The listing builds one solid part. Answer for the finished solid, in the listing's coordinates (mm). A direction names the side the tool comes from. Give positions to 0.01 mm unless a question says otherwise; leave off trailing zeros. Write each loop counter-clockwise with the first axis right and the second up, starting at its lowest first coordinate (ties: lowest second). Pieces come first, ordered by that corner, then holes.
```python
from build123d import *

# Parameters (mm, degrees)
SKETCH2_R           = 20
SKETCH2_R_2         = 10
BOSS_EXTRUDE1_DEPTH = 26
SKETCH3_W           = 50.5
SKETCH3_H           = 100
BOSS_EXTRUDE2_DEPTH = 50
SKETCH6_W           = 19
SKETCH6_H           = 19
CUT_EXTRUDE1_DEPTH  = 129.115426472
CUT_EXTRUDE5_DEPTH  = 105.049267177
CUT_EXTRUDE6_DEPTH  = 105.049267177


with BuildPart() as part:
    # Sketch2 → Boss-Extrude1 (new body)
    with BuildSketch(Plane(origin=(0, 0, 0), x_dir=(0, 0, -1), z_dir=(1, 0, 0))):
        with Locations(Location((0, 0, 0), (0, 0, 180))):
            Circle(SKETCH2_R)
        with Locations(Location((0, 0, 0), (0, 0, 180))):
            Circle(SKETCH2_R_2, mode=Mode.SUBTRACT)
    extrude(amount=BOSS_EXTRUDE1_DEPTH)

    # Sketch3 → Boss-Extrude2 (add)
    with BuildSketch(Plane(origin=(26, 0, 0), x_dir=(0, 0, -1), z_dir=(1, 0, 0))):
        Rectangle(SKETCH3_W, SKETCH3_H)
    extrude(amount=BOSS_EXTRUDE2_DEPTH)

    # Sketch6 → Cut-Extrude1 (cut, through all)
    with BuildSketch(Plane.XZ.offset(50)):
        with Locations((35.5, 0)):
            Rectangle(SKETCH6_W, SKETCH6_H)
    extrude(amount=-CUT_EXTRUDE1_DEPTH, mode=Mode.SUBTRACT)

    # Sketch7 → Cut-Extrude5 (cut, through all)
    with BuildSketch(Plane(origin=(0, 0, -25.25), x_dir=(-1, 0, 0), z_dir=(0, 0, -1))):
        Polygon((-60, 50), (-26, 50), (-26, 35.294942904), align=None)
        Polygon((-60, -50), (-26, -35.294942904), (-26, -50), align=None)
    extrude(amount=-CUT_EXTRUDE5_DEPTH, mode=Mode.SUBTRACT)

    # Sketch9 → Cut-Extrude6 (cut, through all)
    with BuildSketch(Plane(origin=(0, 0, -25.25), x_dir=(-1, 0, 0), z_dir=(0, 0, -1))):
        Polygon((-76, 19.807249774), (-76, -25.192750226), (-61.483507586, -12), (-61.483507586, 12), align=None)
    extrude(amount=-CUT_EXTRUDE6_DEPTH, mode=Mode.SUBTRACT)


solid = part.part
```
Item 1: Each of these flat-tipped pins is pushed along its axis until it touches: P1, Ø4, axis at x = 47.5, z = -3, coming from the +Y side; P2, Ø6, axis at x = 21, y = -13.5, coming from the -Z side; P3, Ø5, axis at x = 43, z = 16, coming from the +Y side. Where does it stop, or does it pass through?
Conclusion:
P1: stops at y = 45.46
P2: stops at z = -17.02
P3: stops at y = 43.73
Item 2: A cutting plane is placed at A-A, the plane z = 0. Give the vertices of the cut face in (x, y).
Conclusion:
outline: (0, -20) - (26, -20) - (26, -10) - (0, -10) - close; (0, 10) - (26, 10) - (26, 20) - (0, 20) - close; (45, -43.51) - (60, -50) - (76, -50) - (76, -25.19) - (61.48, -12) - (61.48, 12) - (76, 19.81) - (76, 50) - (60, 50) - (45, 43.51) - close
Item 3: A cutting plane is placed at C-C, the plane y = 0. Give the vertices of the cut face in (x, z), plus the area to 3 significant figures.
Conclusion:
outline: (0, -20) - (26, -20) - (26, -25.25) - (61.48, -25.25) - (61.48, 25.25) - (26, 25.25) - (26, 20) - (0, 20) - (0, 10) - (26, 10) - (26, 9.5) - (45, 9.5) - (45, -9.5) - (26, -9.5) - (26, -10) - (0, -10) - close
area: 1,950 mm2
Item 4: Determine the mould class of faces 5 (the face through (45, -1, 0)), 6 (the face through (68.64, 15.85, -0.35)), 7 (the face through (68, 50, 0)) for opening direction Y: pulls with the +Y half, pulls with the -Y half, needs draft (parallel to the pull), parting line crosses it, or undercut.
Conclusion:
face 5: needs draft
face 6: undercut
face 7: pulls with the +Y half
Item 5: A cutting plane is placed at B-B, the plane x = 27.5. Give the vertices of the cut face in (y, z), plus the area to 3 significant figures.
Conclusion:
outline: (-35.94, -25.25) - (35.94, -25.25) - (35.94, -9.5) - (-35.94, -9.5) - close; (-35.94, 9.5) - (35.94, 9.5) - (35.94, 25.25) - (-35.94, 25.25) - close
area: 2,260 mm2
Item 6: Consider probe 1 along Y at (x, z) = (13, 0); probe 2 along Z at (x, y) = (42, 39.5); probe 3 along X at (y, z) = (-28.5, 8). Determine where each line is inside the solid, lowest interval first.
Conclusion:
probe 1: y = -20 to -10, 10 to 20
probe 2: z = -25.25 to -9.5, 9.5 to 25.25
probe 3: x = 45 to 76
Item 7: Which of the six approach directions +Z, -Z, +X, -X, +Y, -Y give full straight-line access (tool end or side, diameter ignored) to faces 1 (the face through (61.484, 0, 0)), 2 (the face through (26, 0, -21)), 3 (the face through (13, 0, -10)), 4 (the face through (26, 13, 0))?
Conclusion:
face 1: +Z, -Z, +X
face 2: -Z, -X
face 3: -X
face 4: +Y, -Y
Item 8: A cutting plane is placed at D-D, the plane x = 63. Give the vertices of the cut face in (y, z), plus the area to 3 significant figures.
Conclusion:
outline: (-50, -25.25) - (-13.38, -25.25) - (-13.38, 25.25) - (-50, 25.25) - close; (12.82, -25.25) - (50, -25.25) - (50, 25.25) - (12.82, 25.25) - close
area: 3,730 mm2
